Build history of the part. All positions in model axes, mm. Face numbers are marked on the shaded views. A direction names the side the tool comes from. Round coordinates to 2 decimals unless told otherwise and drop trailing zeros. Write each loop counter-clockwise with the first axis right and the second up, starting at its lowest first coordinate (ties: lowest second). Pieces come first, ordered by that corner, then holes.
1) Saw through at C-C (z = 54.5). Write the cut outline in (x, y), plus the area to 3 significant figures.
2) Saw through at A-A (z = 11.5). Write the cut outline in (x, y).
3) Wall check: probe 1 along Z at (x, y) = (10.5, -6.5); probe 2 along X at (y, z) = (-8, -50); probe 3 along X at (y, z) = (-9.5, 50). Give the ranges that are in metal, low to high.
4) Saw through at B-B (y = -3.5). State how many separate pieces and enclosed holes the cut face has, plus the area to 3 significant figures.
5) Which spindle directions (+Z, -Z, +X, -X, +Y, -Y) get a long thin tool onto all of the face, cutting with end or side? Do the marked faces 4 and 5. Say none if no direction does.
6) Pull direction Z, two halves, no side cores. Call the marked faces 1, 2 and 3: +Z half, -Z half, draft (parallel to the pull), parting line (faces both ways), or undercut.
7) Flat gauge pins, fed straight in: pin 1 (1.6 mm diameter, centred on x = 16, z = -50, fed in from -Y); pin 2 (2 mm diameter, centred on y = -14.5, z = -11, fed in from -X); pin 3 (2 mm diameter, centred on y = -17, z = 3.5, fed in from +X). Where does each tip first touch, or does it go through?
from build123d import *

# Parameters (mm, degrees)
REVOLUTION_ANGLE   = -180
SKETCH002_W        = 30
SKETCH002_H        = 90
POCKET_DEPTH       = 11
HOLE_D             = 1.2
HOLE_DEPTH         = 32
HOLE_CBORE_D       = 3
HOLE_CBORE_DEPTH   = 15
POLARPATTERN_COUNT = 4
FILLET_R           = 2


with BuildPart() as part:
    # Sketch → Revolution (revolve)
    with BuildSketch(Plane.XZ):
        Polygon((10, 80), (11, 50), (11, 0), (21, 0), (21, 50), (15, 80), align=None)
    revolution = revolve(axis=Axis((0, 0, 0), (0, 0, 1)), revolution_arc=REVOLUTION_ANGLE)

    # Mirrored003: Revolution across XY
    add(revolution.mirror(Plane.XY))

    # Sketch002 → Pocket (cut)
    with BuildSketch(Plane.XZ):
        Rectangle(SKETCH002_W, SKETCH002_H)
    extrude(amount=POCKET_DEPTH, mode=Mode.SUBTRACT)

    # Hole
    with Locations(Plane.XZ.offset(20)):
        with Locations((16, 50)):
            hole = CounterBoreHole(HOLE_D / 2, HOLE_CBORE_D / 2, HOLE_CBORE_DEPTH, depth=HOLE_DEPTH)

    # PolarPattern: Hole ×4 about axis
    polarpattern_axis = Axis((0, 0, 0), (0, 1, 0))
    for i in range(1, POLARPATTERN_COUNT):
        add(hole.rotate(polarpattern_axis, i * 360 / POLARPATTERN_COUNT), mode=Mode.SUBTRACT)

    # Mirrored: Hole across XY
    add(hole.mirror(Plane.XY), mode=Mode.SUBTRACT)

    # Mirrored004: Hole across Sketch003 V_Axis
    add(hole.mirror(Plane(origin=(0, -20, 0), x_dir=(0, -1, 0), z_dir=(1, 0, 0))), mode=Mode.SUBTRACT)

    # Fillet
    fillet_edges = [part.edges().sort_by_distance(p)[0] for p in [
        (0, -10, 80),
        (0, -15, 80),
        (0, -10, -80),
        (0, -15, -80),
    ]]
    fillet(fillet_edges, radius=FILLET_R)


solid = part.part
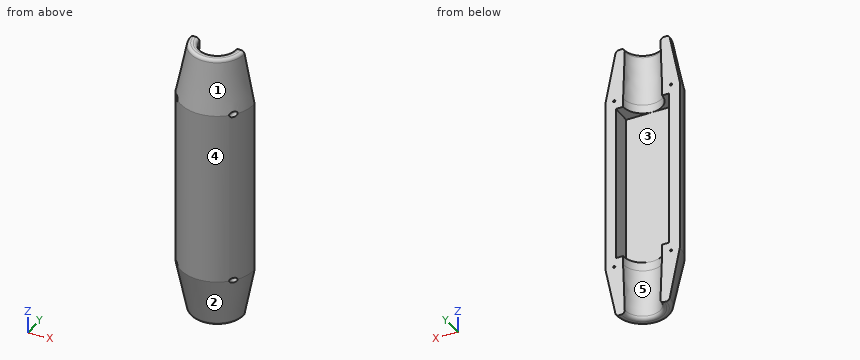
Evaluation:
1. outline: (-20.1, 0) arc R20.1 ccw to (20.1, 0) - (10.85, 0) arc R10.85 cw to (-10.85, 0) - close
1. area: 450 mm2
2. outline: (-21, 0) arc R21 ccw to (21, 0) - (15, 0) - (15, -11) - (-15, -11) - (-15, 0) - close
3. probe 1: z = -80 to -45, 45 to 80
3. probe 2: x = -19.42 to -17.5, -14.5 to -7.55, 7.55 to 14.5, 17.5 to 19.42
3. probe 3: x = -18.73 to -17.5, -14.5 to -5.55, 5.55 to 14.5, 17.5 to 18.73
4. separate pieces: 2
4. enclosed holes: 4
4. area: 2,150 mm2
5. face 4: +Z, -Z, -Y
5. face 5: +Y
6. face 1: +Z half
6. face 2: -Z half
6. face 3: undercut
7. pin 1: stops at y = -5
7. pin 2: stops at x = -16.09
7. pin 3: stops at x = 13.6
